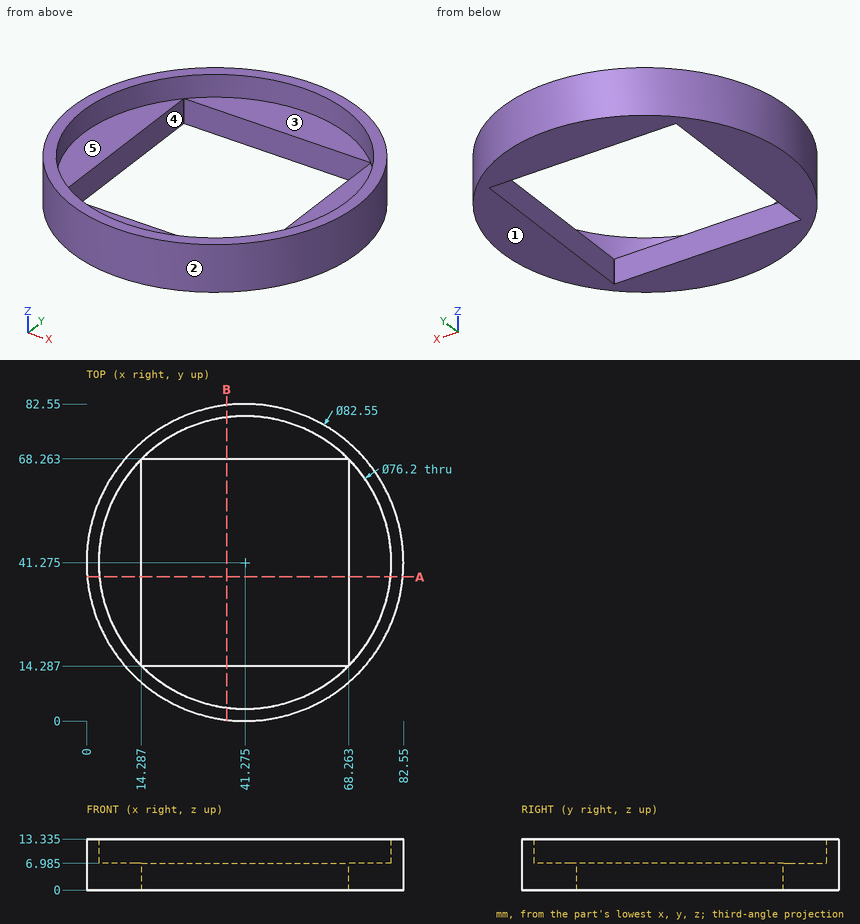
Study the drawing (mm; zero at the part's minimum x, y, z) and answer. A direction names the side the tool comes from. Give positions to 0.01 mm unless a question says otherwise; leave off trailing zeros. Loops run counter-clockwise (first coordinate to the right, second up) from the corner with the lowest first, then second, coordinate; pieces in that order, holes last. Notation, with made-up numbers: (45, 78) -> (68, 78) arc R16 ccw to (68, 107) -> close; hole circle Ø5 at (-18.5, 12.25). An arc over 180 degrees is marked (long way). Write item = value, one per line. Start each with the question number.
(1) Which of the six approach directions +Z, -Z, +X, -X, +Y, -Y give full straight-line access (tool end or side, diameter ignored) to the marked faces 4 and 5?
(2) Given pin 1 Ø9 at (x, y) = (72, 41) entering from +Z (1 decimal); pin 2 Ø8 at (x, z) = (69, 11.5) entering from +Y; pin 3 Ø2 at (y, z) = (52.5, 2) entering from +X, each flat-ended and moving along its own axis, determine where each tip first touches the part or whether it passes through.
(3) Find section A-A on y = 37.5. Give the vertices of the cut face in (x, z) (1 decimal).
(4) Find section B-B on x = 36.5. Give the vertices of the cut face in (y, z) (1 decimal), and give its area (3 significant figures).
(5) Find the intervals of material crossed by probe 1 along Y at (x, z) = (40, 0.5); probe 2 along Y at (x, z) = (46.5, 3.5); probe 3 along X at (y, z) = (51, 9), in increasing order. Write a range as from..to.
(6) The mould has two halves that part along Y. Classify the marked faces 1, 2 and 3: +Y half, -Y half, draft (parallel to the pull), parting line (faces both ways), or undercut.
From the geometry:
q1.face_4 = +Z, -Z
q1.face_5 = +Z
q2.pin_1 = 7
q2.pin_2 = 75.05
q2.pin_3 = 81.26
q3.outline = (0.2, 0) -> (14.3, 0) -> (14.3, 7) -> (3.4, 7) -> (3.4, 13.3) -> (0.2, 13.3) -> close; (68.3, 0) -> (82.4, 0) -> (82.4, 13.3) -> (79.2, 13.3) -> (79.2, 7) -> (68.3, 7) -> close
q4.outline = (0.3, 0) -> (14.3, 0) -> (14.3, 7) -> (3.5, 7) -> (3.5, 13.3) -> (0.3, 13.3) -> close; (68.3, 0) -> (82.3, 0) -> (82.3, 13.3) -> (79.1, 13.3) -> (79.1, 7) -> (68.3, 7) -> close
q4.area = 236 mm^2
q5.probe_1 = 0.02..14.29, 68.26..82.53
q5.probe_2 = 0.33..14.29, 68.26..82.22
q5.probe_3 = 1.16..4.44, 78.11..81.39
q6.face_1 = draft
q6.face_2 = parting line
q6.face_3 = undercut
